Could you check a few things on this model? Use its own coordinates, in mm. Coordinates: 2 decimals unless noted, no trailing zeros. Loops run counter-clockwise (first coordinate to the right, second up) from the corner with the lowest first, then second, coordinate; pieces in that order, holes last. Notation, with made-up numbers: (16, 18) -> (57, 18) arc R20 cw to (57, 29) -> close; hole circle Ø7 at (20.5, 71.25). An arc over 180 degrees is marked (long way). One line per question, with ' | ' between items.
```python
from build123d import *

# Parameters (mm, degrees)
F0_W     = 250
F0_H     = 250
F1_DEPTH = 8
F2_R     = 20
F3_SIZE  = 2.5


with BuildPart() as f1:
    # F0 (on Front) → F1 (new body)
    with BuildSketch(Plane.XZ):
        with Locations((5.8226548135, 13.2943871957)):
            Rectangle(F0_W, F0_H)
    extrude(amount=F1_DEPTH)

    # F2
    f2_edges = [f1.edges().sort_by_distance(p)[0] for p in [
        (-119.177345, -4, -111.705613),
        (130.822655, -4, -111.705613),
        (130.822655, -4, 138.294387),
        (-119.177345, -4, 138.294387),
    ]]
    fillet(f2_edges, radius=F2_R)

    # F3
    f3_edges = [f1.edges().sort_by_distance(p)[0] for p in [
        (5.822655, 0, -111.705613),
        (-113.319481, 0, -105.847748),
        (-119.177345, 0, 13.294387),
        (-113.319481, 0, 132.436523),
        (5.822655, 0, 138.294387),
        (124.96479, 0, 132.436523),
        (124.96479, 0, -105.847748),
        (130.822655, 0, 13.294387),
        (124.96479, -8, -105.847748),
        (5.822655, -8, -111.705613),
    ]]
    chamfer(f3_edges, length=F3_SIZE)


solid = f1.part
```
Q1. Imagine slicing it at A-A on y = -6.75. Write out the boundary of the cut face in (x, z).
Values follow:
outline: (-117.93, -91.71) arc R18.75 ccw to (-99.18, -110.46) -> (110.82, -110.46) arc R18.75 ccw to (129.57, -91.71) -> (129.57, 118.29) arc R18.75 ccw to (110.82, 137.04) -> (-99.18, 137.04) arc R18.75 ccw to (-117.93, 118.29) -> close
Q2. We'd pull the mould along X, two halves only. Please class faces 1 (the face through (-113.474, -4.021, 132.28)), 2 (the face through (123.364, -0.434, -104.526)), 3 (the face through (4, -8, 15)): released by +X, released by -X, zero draft, split by the parting line, or undercut.
Values follow:
face 1: released by -X | face 2: released by +X | face 3: zero draft
Q3. Please list where these lines run through material, in increasing order: L1, parallel to Z at x = 112.5, y = -4; L2, parallel to X at y = -7.25, z = -45; L3, parallel to Z at x = -34.5, y = -6.75. Write a range as [from, to].
Values follow:
L1: z = [-111.64, 138.22] | L2: x = [-117.43, 129.07] | L3: z = [-110.46, 137.04]
